Here's how the part is built. I have some questions about the finished solid (model axes, mm). A direction names the side the tool comes from. Give positions to 0.01 mm unless a question says otherwise; leave off trailing zeros. Loops run counter-clockwise (first coordinate to the right, second up) from the corner with the lowest first, then second, coordinate; pieces in that order, holes last. Notation, with made-up numbers: (84, 80.5) -> (136, 80.5) arc R5 cw to (136, 86.5) -> close; hole circle Ø11 at (44, 23.25). An arc over 180 degrees is marked (long way). Answer in a Markdown table with one row per item. Add a question column.
Item 1: If we section it at B-B (z = -25.5): Write out the boundary of the cut face in (x, y).
Item 2: For P1, Ø6, axis at x = 4.5, z = 9.5, coming from the -Y side; P2, Ø6, axis at y = -3, z = 8, coming from the +X side; P3, Ø3, axis at y = 3.5, z = 18.5, coming from the -X side, each with a flat end and sliding along its axis, tell me the tip position at first contact or that it passes through.
Item 3: We'd pull the mould along Z, two halves only. Please class faces 1 (the face through (-0.77, 3.45, -56.42)), 2 (the face through (-4, 2, -60)), 3 (the face through (1.535, 0.483, 83.091)): released by +Z, released by -Z, zero draft, split by the parting line, or undercut.
Item 4: Which directions (+Z, -Z, +X, -X, +Y, -Y) give clear straight access to the entire face, cutting with the end or side of a thin tool? Please do faces 4 (the face through (2.5, 2.5, -55)), 5 (the face through (0, 0, -55)), 6 (the face through (-2.17, 1.664, 72.395)), 7 (the face through (6.383, 2.01, 47.395)).
Item 5: If I drill on line 1 (X direction, y = 0.5, z = 1); line 2 (Z direction, x = -2.75, y = 3); line 3 (Y direction, x = 0.25, z = -39.5), over which ranges is the centre line in solid material (lowest first)?
Item 6: If we section it at A-A (z = 43.5): Write out the boundary of the cut face in (x, y), then the cut area to 3 significant figures.
```python
from build123d import *

# Parameters (mm, degrees)
F0_R          = 6.6693816334
F1_DEPTH      = 5
F1_DEPTH_BACK = 50
F1_FACE_R     = 6.6693816334
F2_DEPTH      = 5
F2_TAPER      = 10
F1_FACE1_R    = 6.6693816334
F3_DEPTH      = 5
F3_TAPER      = 10
F4_R          = 3.0163554994
F5_DEPTH      = 5
F5_TAPER      = -20
F6_R          = 4.3040236216
F7_DEPTH      = 5
F7_TAPER      = 20
F8_DEPTH      = 30
F9_R          = 6.6922824671
F10_DEPTH     = 15
F10_FACE_R    = 6.6922824671
F11_DEPTH     = 5
F11_TAPER     = 10
F11_FACE_R    = 5.8106475635
F12_DEPTH     = 3
F12_TAPER     = 13
F12_FACE_R    = 5.1180429902
F13_DEPTH     = 2
F13_TAPER     = 50
F14_DEPTH     = 15
F14_FACE_R    = 2.734535805
F15_DEPTH     = 5
F15_TAPER     = 20


with BuildPart() as f1:
    # F0 (on Top) → F1 (new body, two sides)
    with BuildSketch(Plane.XY) as f1_sk:
        Circle(F0_R)
    extrude(amount=F1_DEPTH)
    extrude(f1_sk.sketch, amount=-F1_DEPTH_BACK)

    # F1_face (on face) → F2 (join)
    with BuildSketch(Plane.XY.offset(5)):
        Circle(F1_FACE_R)
    extrude(amount=F2_DEPTH, taper=F2_TAPER)

    # F1_face1 (on face) → F3 (join)
    with BuildSketch(Plane(origin=(0, 0, -50), x_dir=(1, 0, 0), z_dir=(0, 0, -1))):
        Circle(F1_FACE1_R)
    extrude(amount=F3_DEPTH, taper=F3_TAPER)

    # F4 (on face) → F5 (join)
    with BuildSketch(Plane(origin=(0, 0, -55), x_dir=(1, 0, 0), z_dir=(0, 0, -1))):
        Circle(F4_R)
    extrude(amount=F5_DEPTH, taper=F5_TAPER)

    # F6 (on face) → F7 (cut)
    with BuildSketch(Plane(origin=(0, 0, -60), x_dir=(1, 0, 0), z_dir=(0, 0, -1))):
        Circle(F6_R)
    extrude(amount=-F7_DEPTH, taper=F7_TAPER, mode=Mode.SUBTRACT)

    # F8 (add): a face of the model
    f8_faces = [f1.faces().sort_by_distance(p)[0] for p in [
        (0, 0, 10),
    ]]
    extrude(f8_faces, amount=F8_DEPTH)

    # F9 (on face) → F10 (join)
    with BuildSketch(Plane.XY.offset(40)):
        Circle(F9_R)
    extrude(amount=F10_DEPTH)

    # F10_face (on face) → F11 (join)
    with BuildSketch(Plane.XY.offset(55)):
        Circle(F10_FACE_R)
    extrude(amount=F11_DEPTH, taper=F11_TAPER)

    # F11_face (on face) → F12 (join)
    with BuildSketch(Plane.XY.offset(60)):
        Circle(F11_FACE_R)
    extrude(amount=F12_DEPTH, taper=F12_TAPER)

    # F12_face (on face) → F13 (join)
    with BuildSketch(Plane.XY.offset(63)):
        Circle(F12_FACE_R)
    extrude(amount=F13_DEPTH, taper=F13_TAPER)

    # F14 (add): a face of the model
    f14_faces = [f1.faces().sort_by_distance(p)[0] for p in [
        (0, 0, 65),
    ]]
    extrude(f14_faces, amount=F14_DEPTH)

    # F14_face (on face) → F15 (join)
    with BuildSketch(Plane.XY.offset(80)):
        Circle(F14_FACE_R)
    extrude(amount=F15_DEPTH, taper=F15_TAPER)


solid = f1.part
```
Recorded:
| question | item | result |
|---|---|---|
| 1 | outline | circle Ø13.34 at (0, 0) |
| 2 | P1 | stops at y = -5.84 |
| 2 | P2 | stops at x = 6.46 |
| 2 | P3 | stops at x = -5.43 |
| 3 | face 1 | undercut |
| 3 | face 2 | released by -Z |
| 3 | face 3 | released by +Z |
| 4 | face 4 | none |
| 4 | face 5 | -Z |
| 4 | face 6 | +Z |
| 4 | face 7 | +Z, -Z |
| 5 | line 1 | x = -6.65 to 6.65 |
| 5 | line 2 | z = -59.36 to -57.89, -55 to 63.88 |
| 5 | line 3 | y = -6.66 to 6.66 |
| 6 | outline | circle Ø13.38 at (0, 0) |
| 6 | area | 141 mm^2 |
